from build123d import *

# Parameters (mm, degrees)
BOSS_EXTRUDE1_DEPTH = 31.5
BOSS_EXTRUDE2_START = -31.5
SKETCH2_W           = 2
SKETCH2_H           = 1.6
BOSS_EXTRUDE2_DEPTH = 1


with BuildPart() as part:
    # Sketch1 → Boss-Extrude1 (new body)
    with BuildSketch(Plane.XY):
        with BuildLine():
            Line((-1.9, 5.8), (-0.9, 5.8))
            ThreePointArc((-0.9, 5.8), (0, 6.7), (0.9, 5.8))
            Line((0.9, 5.8), (2, 5.8))
            Line((2, 5.8), (2, 0.8))
            Line((2, 0.8), (0, 0.8))
            Line((0, 0.8), (0, -0.8))
            Line((0, -0.8), (2, -0.8))
            Line((2, -0.8), (2, -5.8))
            Line((2, -5.8), (0.90202041, -5.8))
            ThreePointArc((0.90202041, -5.8), (0.00202041, -6.7), (-0.89797959, -5.8))
            Line((-0.89797959, -5.8), (-1.9, -5.8))
            Line((-1.9, -5.8), (-1.9, 5.8))
        make_face()
    extrude(amount=BOSS_EXTRUDE1_DEPTH)

    # Sketch2 → Boss-Extrude2 (add)
    with BuildSketch(Plane(origin=(0, 0, 0), x_dir=(-1, 0, 0), z_dir=(0, 0, -1)).offset(BOSS_EXTRUDE2_START)):
        with Locations((-1, 0)):
            Rectangle(SKETCH2_W, SKETCH2_H)
    extrude(amount=BOSS_EXTRUDE2_DEPTH)


solid = part.part
Check sheet for the modelled part. Datum: model origin and axes. Units: mm. A direction names the side the tool comes from. Give positions to 0.01 mm unless a question says otherwise; leave off trailing zeros. Order: outer loops, then holes, each group sorted by start corner. A loop starts at its lowest first (then second) coordinate and runs counter-clockwise, first axis right, second up. Notation, with made-up numbers: M 21.5,57.5 L 66.5,57.5 A11 ccw 66.5,64.5 Z; hole C 48,50 d8. An arc over 180 degrees is marked long. Answer as CSV lines item,"result". Start each with the question number.
Item 1: Cross-section at C-C on y = -0.25. Enter the section's corners in (x, z), plus the area to 4 significant figures.
Item 2: Gauge pin test, flat ends, axial feed: P1, Ø0.6, axis at x = 1.5, z = 17.5, coming from the +Y side; P2, Ø1.6, axis at x = 1, z = 10, coming from the -Y side. Record the tip position at first contact, or that the pin passes through.
Item 3: Tool access check on faces 1 (the face through (1, 0, 30.5)), 2 (the face through (-1.4, -5.8, 15.5)), 3 (the face through (1.5, -5.8, 15.5)), 4 (the face through (1.4, 5.8, 15.5)). Record the directions out of +Z, -Z, +X, -X, +Y, -Y that give a thin tool (end or side, any length) a straight path to the whole face; none if there is none.
Item 4: Cross-section at B-B on z = 2.5. Enter the section's corners in (x, y), plus the area to 3 significant figures.
Item 5: Thickness scan on line 1 (X direction, y = -0.5, z = 9); line 2 (Y direction, x = 0.15, z = 14); line 3 (Y direction, x = -1.2, z = 22). Record the ranges inside material, lowest first. Write a range as [from, to].
Item 6: Mould release check, pull along Y, two halves, no side actions. Record for faces 5 (the face through (0, 0, 31.5)), 6 (the face through (-1.4, 5.8, 15.5)), 7 (the face through (0, 0, 15)): +Y half, -Y half, draft (parallel to the pull), parting line (faces both ways), or undercut.
Item 7: Cross-section at A-A on x = 1.55. Enter the section's corners in (y, z), plus the area to 3 significant figures.
Item 8: Cross-section at D-D on x = -1.45. Enter the section's corners in (y, z), plus the area to 3 significant figures.
Established:
1,outline,"M -1.9,0 L 0,0 L 0,30.5 L 2,30.5 L 2,31.5 L -1.9,31.5 Z"
1,area,"61.85 mm^2"
2,P1,"stops at y = 5.8"
2,P2,"stops at y = -6.68"
3,face 1,"-Z, +X"
3,face 2,"+Z, -Z, -X, -Y"
3,face 3,"+Z, -Z, +X, -Y"
3,face 4,"+Z, -Z, +X, +Y"
4,outline,"M -1.9,-5.8 L -0.9,-5.8 A0.9 ccw 0.9,-5.8 L 2,-5.8 L 2,-0.8 L 0,-0.8 L 0,0.8 L 2,0.8 L 2,5.8 L 0.9,5.8 A0.9 ccw -0.9,5.8 L -1.9,5.8 Z"
4,area,"44.6 mm^2"
5,line 1,"x = [-1.9, 0]"
5,line 2,"y = [-6.69, -0.8], [0.8, 6.69]"
5,line 3,"y = [-5.8, 5.8]"
6,face 5,"draft"
6,face 6,"+Y half"
6,face 7,"undercut"
7,outline,"M -5.8,0 L -0.8,0 L -0.8,30.5 L 0.8,30.5 L 0.8,0 L 5.8,0 L 5.8,31.5 L -5.8,31.5 Z"
7,area,"317 mm^2"
8,outline,"M -5.8,0 L 5.8,0 L 5.8,31.5 L -5.8,31.5 Z"
8,area,"365 mm^2"
